```python
from build123d import *

# Parameters (mm, degrees)
EXTRUDE_2007_DEPTH      = 5
FILLET_3_R              = 1.5
FILLET_4_R              = 1.5
FILLET_5_R              = 1.5
FILLET_6_R              = 1.5
FILLET_8_R              = 1.5
FILLET_9_R              = 1.5
FILLET_10_R             = 1
SKETCH_3_R              = 17
EXTRUDE_3379_DEPTH      = 45
SKETCH_4_R              = 15.5
CUT_EXTRUDE_3486_DEPTH  = 45
SKETCH_5_R              = 1.5
CUT_EXTRUDE_4485_DEPTH  = 2
SKETCH_12_R             = 3.5
CUT_EXTRUDE_5429_DEPTH  = 3
CUT_EXTRUDE_START       = -3.5
CUT_EXTRUDE_6212_DEPTH  = 3.5
SKETCH_8_W              = 26
SKETCH_8_H              = 49
CUT_EXTRUDE_6714_DEPTH  = 5
SKETCH_9_R              = 1.5
CUT_EXTRUDE_7323_DEPTH  = 2
SKETCH_10_R             = 3.5
CUT_EXTRUDE_8111_DEPTH  = 3
SKETCH_11_R             = 1.5
CUT_EXTRUDE_8692_DEPTH  = 5
SKETCH_14_W             = 68
SKETCH_14_H             = 4
CUT_EXTRUDE_1_DEPTH     = 10
SKETCH_15_R             = 1.5
CUT_EXTRUDE_9738_DEPTH  = 134.667497919
SKETCH_16_R             = 1.5
CUT_EXTRUDE_10559_DEPTH = 10


with BuildPart() as part:
    # 草图1 → Extrude 2007 (new body)
    with BuildSketch(Plane.XY):
        with BuildLine():
            Line((40.60409347, 62.431357903), (55.904485703, 42.127051621))
            Line((55.904485703, 42.127051621), (70.756031924, 22.418384115))
            ThreePointArc((70.756031924, 22.418384115), (72.202279258, 21.378104776), (73.983419946, 21.341358278))
            Line((73.983419946, 21.341358278), (85.513303574, 24.667284243))
            ThreePointArc((85.513303574, 24.667284243), (88.605814226, -8.36717906), (79.384125876, -40.238794203))
            Line((79.384125876, -40.238794203), (70.659905832, -35.816599072))
            ThreePointArc((70.659905832, -35.816599072), (69.012874234, -35.506582977), (67.456557556, -36.128436223))
            Line((67.456557556, -36.128436223), (43.096303273, -55.160752752))
            Line((43.096303273, -55.160752752), (24.916466517, -69.364397902))
            ThreePointArc((24.916466517, -69.364397902), (23.892889166, -70.856722021), (23.91379502, -72.666226046))
            Line((23.91379502, -72.666226046), (27.821277866, -84.539792393))
            ThreePointArc((27.821277866, -84.539792393), (0, -89), (-27.821277866, -84.539792393))
            Line((-27.821277866, -84.539792393), (-23.91379502, -72.666226046))
            ThreePointArc((-23.91379502, -72.666226046), (-23.892889166, -70.856722021), (-24.916466517, -69.364397902))
            Line((-24.916466517, -69.364397902), (-43.096303273, -55.160752752))
            Line((-43.096303273, -55.160752752), (-67.456557556, -36.128436223))
            ThreePointArc((-67.456557556, -36.128436223), (-69.012874234, -35.506582977), (-70.659905832, -35.816599072))
            Line((-70.659905832, -35.816599072), (-79.384125876, -40.238794203))
            ThreePointArc((-79.384125876, -40.238794203), (-88.605814226, -8.36717906), (-85.513303574, 24.667284243))
            Line((-85.513303574, 24.667284243), (-73.983419946, 21.341358278))
            ThreePointArc((-73.983419946, 21.341358278), (-72.202279258, 21.378104776), (-70.756031924, 22.418384115))
            Line((-70.756031924, 22.418384115), (-55.904485703, 42.127051621))
            Line((-55.904485703, 42.127051621), (-40.60409347, 62.431357903))
            ThreePointArc((-40.60409347, 62.431357903), (-40.155029034, 63.284889003), (-40, 64.236802972))
            Line((-40, 64.236802972), (-40, 74))
            Line((-40, 74), (-40, 80.06403687))
            Line((-40, 80.06403687), (-34, 82.790397994))
            Line((-34, 82.790397994), (-34, 77))
            Line((-34, 77), (34, 77))
            Line((34, 77), (34, 82.790397994))
            Line((34, 82.790397994), (40, 80.06403687))
            Line((40, 80.06403687), (40, 74))
            Line((40, 74), (40, 64.236802972))
            ThreePointArc((40, 64.236802972), (40.155029034, 63.284889003), (40.60409347, 62.431357903))
        make_face()
    extrude(amount=EXTRUDE_2007_DEPTH)

    # 圆角3
    fillet_3_edges = [part.edges().sort_by_distance(p)[0] for p in [
        (79.384125876, -40.238794203, 2.5),
    ]]
    fillet(fillet_3_edges, radius=FILLET_3_R)

    # 圆角4
    fillet_4_edges = [part.edges().sort_by_distance(p)[0] for p in [
        (27.821277866, -84.539792393, 2.5),
    ]]
    fillet(fillet_4_edges, radius=FILLET_4_R)

    # 圆角5
    fillet_5_edges = [part.edges().sort_by_distance(p)[0] for p in [
        (-27.821277866, -84.539792393, 2.5),
    ]]
    fillet(fillet_5_edges, radius=FILLET_5_R)

    # 圆角6
    fillet_6_edges = [part.edges().sort_by_distance(p)[0] for p in [
        (-79.384125876, -40.238794203, 2.5),
    ]]
    fillet(fillet_6_edges, radius=FILLET_6_R)

    # 圆角8
    fillet_8_edges = [part.edges().sort_by_distance(p)[0] for p in [
        (85.513303574, 24.667284243, 2.5),
    ]]
    fillet(fillet_8_edges, radius=FILLET_8_R)

    # 圆角9
    fillet_9_edges = [part.edges().sort_by_distance(p)[0] for p in [
        (-85.513303574, 24.667284243, 2.5),
    ]]
    fillet(fillet_9_edges, radius=FILLET_9_R)

    # 圆角10
    fillet_10_edges = [part.edges().sort_by_distance(p)[0] for p in [
        (-40, 80.06403687, 2.5),
        (-34, 82.790397994, 2.5),
        (34, 82.790397994, 2.5),
        (40, 80.06403687, 2.5),
    ]]
    fillet(fillet_10_edges, radius=FILLET_10_R)

    # 草图3 → Extrude 3379 (add)
    with BuildSketch(Plane.XY.offset(5)):
        with Locations(Location((70, -9.25, 0), (0, 0, 180))):
            Circle(SKETCH_3_R)
    extrude_3379 = extrude(amount=EXTRUDE_3379_DEPTH)

    # 草图4 → Cut-Extrude 3486 (cut)
    with BuildSketch(Plane.XY.offset(50)):
        with Locations((70, -9.25)):
            Circle(SKETCH_4_R)
    cut_extrude_3486 = extrude(amount=-CUT_EXTRUDE_3486_DEPTH, mode=Mode.SUBTRACT)

    # 镜向1: Extrude 3379 across plane
    add(extrude_3379.mirror(Plane(origin=(0, 0, 0), x_dir=(0, 0, 1), z_dir=(1, 0, 0))))

    # 镜向2: Cut-Extrude 3486 across plane
    add(cut_extrude_3486.mirror(Plane(origin=(0, 0, 0), x_dir=(0, 0, 1), z_dir=(1, 0, 0))), mode=Mode.SUBTRACT)

    # 草图5 → Cut-Extrude 4485 (cut)
    with BuildSketch(Plane.XY.offset(5)):
        with Locations((46.888613918, 49.106597162)):
            Circle(SKETCH_5_R)
        with Locations((67.952139729, 21.15435431)):
            Circle(SKETCH_5_R)
        with Locations(Location((-67.952139729, 21.15435431, 0), (0, 0, 180))):
            Circle(SKETCH_5_R)
        with Locations(Location((-46.888613918, 49.106597162, 0), (0, 0, 180))):
            Circle(SKETCH_5_R)
        with Locations((60.161576933, -38.020845084)):
            Circle(SKETCH_5_R)
        with Locations((32.581200557, -59.56899672)):
            Circle(SKETCH_5_R)
        with Locations(Location((-60.161576933, -38.020845084, 0), (0, 0, 180))):
            Circle(SKETCH_5_R)
        with Locations(Location((-32.581200557, -59.56899672, 0), (0, 0, 180))):
            Circle(SKETCH_5_R)
    extrude(amount=-CUT_EXTRUDE_4485_DEPTH, mode=Mode.SUBTRACT)

    # 草图12 → Cut-Extrude 5429 (cut)
    with BuildSketch(Plane(origin=(0, 0, 0), x_dir=(-1, 0, 0), z_dir=(0, 0, -1))):
        with Locations((46.888613918, 49.106597162)):
            Circle(SKETCH_12_R)
        with Locations((68.553954752, 20.3557188)):
            Circle(SKETCH_12_R)
        with Locations((-68.553954752, 20.3557188)):
            Circle(SKETCH_12_R)
        with Locations((-46.888613918, 49.106597162)):
            Circle(SKETCH_12_R)
        with Locations((32.581200557, -59.56899672)):
            Circle(SKETCH_12_R)
        with Locations((60.161576933, -38.020845084)):
            Circle(SKETCH_12_R)
        with Locations((13.527038551, -115.928745256)):
            Circle(SKETCH_12_R)
        with Locations((-60.161576933, -38.020845084)):
            Circle(SKETCH_12_R)
        with Locations((-32.581200557, -59.56899672)):
            Circle(SKETCH_12_R)
    extrude(amount=-CUT_EXTRUDE_5429_DEPTH, mode=Mode.SUBTRACT)

    # 草图7 → Cut-Extrude 6212 (cut)
    with BuildSketch(Plane.XY.offset(5).offset(CUT_EXTRUDE_START)):
        with BuildLine():
            Line((-8, 77), (-8, -88.639720216))
            ThreePointArc((-8, -88.639720216), (0, -89), (8, -88.639720216))
            Line((8, -88.639720216), (8, 77))
            Line((8, 77), (-8, 77))
        make_face()
    extrude(amount=CUT_EXTRUDE_6212_DEPTH, mode=Mode.SUBTRACT)

    # 草图8 → Cut-Extrude 6714 (cut)
    with BuildSketch(Plane.XY.offset(5)):
        with Locations((0, 10.5)):
            Rectangle(SKETCH_8_W, SKETCH_8_H)
    extrude(amount=-CUT_EXTRUDE_6714_DEPTH, mode=Mode.SUBTRACT)

    # 草图9 → Cut-Extrude 7323 (cut)
    with BuildSketch(Plane.XY.offset(5)):
        with Locations((12, 39)):
            Circle(SKETCH_9_R)
        with Locations(Location((-12, 39, 0), (0, 0, 180))):
            Circle(SKETCH_9_R)
        with Locations((-12, -18)):
            Circle(SKETCH_9_R)
        with Locations(Location((12, -18, 0), (0, 0, 180))):
            Circle(SKETCH_9_R)
    extrude(amount=-CUT_EXTRUDE_7323_DEPTH, mode=Mode.SUBTRACT)

    # 草图10 → Cut-Extrude 8111 (cut)
    with BuildSketch(Plane(origin=(0, 0, 0), x_dir=(-1, 0, 0), z_dir=(0, 0, -1))):
        with Locations((12, 39)):
            Circle(SKETCH_10_R)
        with Locations(Location((-12, 39, 0), (0, 0, 180))):
            Circle(SKETCH_10_R)
        with Locations(Location((12, -18, 0), (0, 0, 180))):
            Circle(SKETCH_10_R)
        with Locations((-12, -18)):
            Circle(SKETCH_10_R)
    extrude(amount=-CUT_EXTRUDE_8111_DEPTH, mode=Mode.SUBTRACT)

    # 草图11 → Cut-Extrude 8692 (cut)
    with BuildSketch(Plane.XY.offset(5)):
        with Locations((22.5, 68.8)):
            Circle(SKETCH_11_R)
        with Locations((22.5, 53.8)):
            Circle(SKETCH_11_R)
        with Locations(Location((-22.5, 53.8, 0), (0, 0, 180))):
            Circle(SKETCH_11_R)
        with Locations(Location((-22.5, 68.8, 0), (0, 0, 180))):
            Circle(SKETCH_11_R)
    extrude(amount=-CUT_EXTRUDE_8692_DEPTH, mode=Mode.SUBTRACT)

    # 草图14 → 切除-拉伸1 (cut)
    with BuildSketch(Plane(origin=(0, 0, 0), x_dir=(-1, 0, 0), z_dir=(0, 0, -1))):
        with Locations((0, 75)):
            Rectangle(SKETCH_14_W, SKETCH_14_H)
    extrude(amount=-CUT_EXTRUDE_1_DEPTH, mode=Mode.SUBTRACT)

    # 草图15 → Cut-Extrude 9738 (cut, through all)
    with BuildSketch(Plane.XY.offset(5)):
        with Locations(Location((-45, -12.5, 0), (0, 0, 180))):
            Circle(SKETCH_15_R)
        with Locations(Location((-38, 49, 0), (0, 0, 180))):
            Circle(SKETCH_15_R)
        with Locations((38, 49)):
            Circle(SKETCH_15_R)
        with Locations((45, -12.5)):
            Circle(SKETCH_15_R)
    extrude(amount=-CUT_EXTRUDE_9738_DEPTH, mode=Mode.SUBTRACT)

    # 草图16 → Cut-Extrude 10559 (cut)
    with BuildSketch(Plane.XY.offset(5)):
        with Locations((-70.6, -32.2)):
            Circle(SKETCH_16_R)
        with Locations((-70.6, 10)):
            Circle(SKETCH_16_R)
        with Locations((70.6, 10)):
            Circle(SKETCH_16_R)
        with Locations((70.6, -32.2)):
            Circle(SKETCH_16_R)
    extrude(amount=-CUT_EXTRUDE_10559_DEPTH, mode=Mode.SUBTRACT)


solid = part.part
```
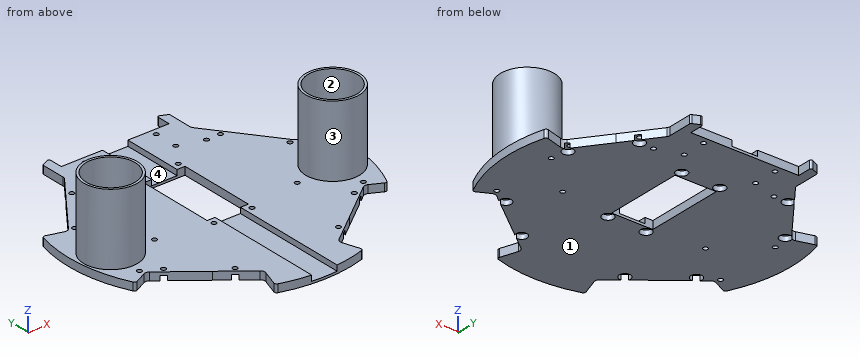
For this review, take the finished solid that the model builds, in its own axes (mm). Face numbers are marked on the shaded views. A direction names the side the tool comes from. Coordinates: 2 decimals unless noted, no trailing zeros. Loops run counter-clockwise (first coordinate to the right, second up) from the corner with the lowest first, then second, coordinate; pieces in that order, holes last.
1. Add section B-B, the plane x = 76. Give the boundary of the cut face in (y, z), then the cut area to 3 significant figures.
2. For line 1 (Y direction, x = 70.5, z = 28.5); line 2 (X direction, y = 55, z = 4); line 3 (Y direction, x = -22, z = 1), list the stretches that pass through material, from the lowest coordinate up.
3. Mouldability with a two-part tool opening along X and no side actions: class the marked faces 1 and 2 as +X half, -X half, draft (parallel to the pull), parting line (faces both ways), or undercut.
4. Add section A-A, the plane z = 12.5. Give the boundary of the cut face in (x, y), then the cut area to 3 significant figures.
5. For the marked faces 3 and 4, list the 3-axis set-ups (+Z, -Z, +X, -X, +Y, -Y) from which the entire face can be reached by the end or side of a thin tool; tool diameter is ignored.
6. Insertion check: P1, Ø2, axis at x = 61, y = -36.5, coming from the -Z side; P2, Ø8, axis at x = 32.58, y = -59.57, coming from the -Z side; P3, Ø5, axis at x = -69.5, y = -35, coming from the +Z side; P4, Ø10, axis at y = -46.5, z = 8.5, coming from the -X side. Each pin has a flat end and moves straight along its axis. Give the tip position at first contact, or say it passes through.
Result:
1. outline: (-38.52, 0) - (21.92, 0) - (21.92, 5) - (6.66, 5) - (6.66, 50) - (5.04, 50) - (5.04, 5) - (-23.54, 5) - (-23.54, 50) - (-25.16, 50) - (-25.16, 5) - (-38.52, 5) - close
1. area: 448 mm2
2. line 1: y = -26.24 to -24.74, 6.24 to 7.74
2. line 2: x = -46.2 to -23.4, -21.6 to -8, 8 to 21.6, 23.4 to 46.2
2. line 3: y = -86.24 to 52.39, 55.21 to 67.39, 70.21 to 73
3. face 1: draft
3. face 2: undercut
4. outline: circle Ø34 at (-70, -9.25); circle Ø34 at (70, -9.25); hole circle Ø31 at (-70, -9.25); hole circle Ø31 at (70, -9.25)
4. area: 306 mm2
5. face 3: +Z
5. face 4: +Z, +Y, -Y
6. P1: stops at z = 3
6. P2: stops at z = 0
6. P3: stops at z = 5
6. P4: stops at x = -58.75
